from build123d import *

# Parameters (mm, degrees)
CUT_EXTRUDE1_DEPTH = 1.3462


with BuildPart() as part:
    # Sketch1 → Revolve1 (revolve)
    with BuildSketch(Plane.XY, mode=Mode.PRIVATE) as revolve1_sk:
        with BuildLine():
            Line((0, 12.7127), (0, 0))
            Line((0, 0), (0.8382, 0))
            Line((0.8382, 0), (1.0922, 0.254))
            Line((1.0922, 0.254), (1.0922, 11.1125))
            Line((1.0922, 11.1125), (2.1209, 11.1125))
            Line((2.1209, 11.1125), (2.1209, 11.9126))
            ThreePointArc((2.1209, 11.9126), (1.133399402, 12.506023812), (0, 12.7127))
        make_face()
    revolve(revolve1_sk.sketch.rotate(Axis((0, 0, 0), (0, 1, 0)), 90), axis=Axis((0, 0, 0), (0, 1, 0)))

    # Sketch2 → Cut-Extrude1 (cut)
    with BuildSketch(Plane(origin=(0, 12.7127, 0), x_dir=(1, 0, 0), z_dir=(0, 1, 0))):
        Polygon((-0.3937, 0.3937), (-0.3937, 1.2192), (0.3937, 1.2192), (0.3937, 0.3937), (1.2192, 0.3937), (1.2192, -0.3937), (0.3937, -0.3937), (0.3937, -1.2192), (-0.3937, -1.2192), (-0.3937, -0.3937), (-1.2192, -0.3937), (-1.2192, 0.3937), align=None)
    extrude(amount=-CUT_EXTRUDE1_DEPTH, mode=Mode.SUBTRACT)


solid = part.part
Geometry check sheet. Reference: the model listing, model coordinates, mm. A direction names the side the tool comes from. Give positions to 0.01 mm unless a question says otherwise; leave off trailing zeros. Write each loop counter-clockwise with the first axis right and the second up, starting at its lowest first coordinate (ties: lowest second). Pieces come first, ordered by that corner, then holes. Notation, with made-up numbers: M 69.5,42 L 125.5,42 A7 cw 125.5,54 Z; hole C 74.5,-4.5 d5. An arc over 180 degrees is marked long. Answer as CSV lines item,"result". Start each with the question number.
Q1. Section check C-C, the plane x = 0. Record the cut outline in (y, z).
Q2. Section check D-D, the plane y = 7.25. Record the cut outline in (x, z).
Q3. Section check B-B, the plane z = 0. Record the cut outline in (x, y).
Q4. Section check A-A, the plane y = 11.5. Record the cut outline in (x, z).
Q5. Go/stop test with flat-tipped pins: pin 1 (1.5 mm diameter, centred on x = -1, y = 4.5, fed in from +Z); pin 2 (0.9 mm diameter, centred on y = 12.5, z = 1, fed in from +X); pin 3 (0.9 mm diameter, centred on x = -1, y = 12, fed in from +Z). Record where each tip stops, or that it passes through.
Q6. Material ranges on L1, parallel to X at y = 9, z = 0.7; L2, parallel to Z at x = -0.6, y = 11.5; L3, parallel to Y at x = 0.3, z = -0.5, recorded low to high.
Q7. Release check for a two-part mould opening along X. For faces 1 (the face through (1, 12, -0.394)), 2 (the face through (-1, 12, 0.394)), 3 (the face through (-0.33, 5.76, -1.04)), 4 (the face through (-1, 11.112, -1)) record: pulls with the +X half, pulls with the -X half, needs draft (parallel to the pull), parting line crosses it, or undercut.
Q8. Tool access check on faces 5 (the face through (2.07, 11.52, 0.46)), 6 (the face through (-1, 12, -0.394)). Record the directions out of +Z, -Z, +X, -X, +Y, -Y that give a thin tool (end or side, any length) a straight path to the whole face; none if there is none.
Geometry says:
1,outline,"M 0,-0.84 L 0.25,-1.09 L 11.11,-1.09 L 11.11,-2.12 L 11.91,-2.12 A3.21 ccw 12.47,-1.22 L 11.37,-1.22 L 11.37,1.22 L 12.47,1.22 A3.21 ccw 11.91,2.12 L 11.11,2.12 L 11.11,1.09 L 0.25,1.09 L 0,0.84 Z"
2,outline,"C 0,0 d2.18"
3,outline,"M -2.12,11.11 L -1.09,11.11 L -1.09,0.25 L -0.84,0 L 0.84,0 L 1.09,0.25 L 1.09,11.11 L 2.12,11.11 L 2.12,11.91 A3.21 ccw 1.22,12.47 L 1.22,11.37 L -1.22,11.37 L -1.22,12.47 A3.21 ccw -2.12,11.91 Z"
4,outline,"C 0,0 d4.24; hole M -1.22,-0.39 L -0.39,-0.39 L -0.39,-1.22 L 0.39,-1.22 L 0.39,-0.39 L 1.22,-0.39 L 1.22,0.39 L 0.39,0.39 L 0.39,1.22 L -0.39,1.22 L -0.39,0.39 L -1.22,0.39 Z"
5,pin 1,"z = 1.06"
5,pin 2,"x = 1.72"
5,pin 3,"z = 2.05"
6,L1,"-0.84 to 0.84"
6,L2,"-2.03 to -0.39, 0.39 to 2.03"
6,L3,"0 to 11.37"
7,face 1,"undercut"
7,face 2,"undercut"
7,face 3,"parting line crosses it"
7,face 4,"needs draft"
8,face 5,"+Y, -Y"
8,face 6,"+Y"
